Geometry: final body of the model. Coordinates: model frame, mm. Give positions to 0.01 mm unless a question says otherwise; leave off trailing zeros. Write each loop counter-clockwise with the first axis right and the second up, starting at its lowest first coordinate (ties: lowest second). Pieces come first, ordered by that corner, then holes.
Q1. Line query: line 1 (X direction, y = 195, z = 2); line 2 (X direction, y = 263.5, z = 4.75); line 3 (Y direction, x = 144.5, z = 3.25). Output: solid intervals per line, ascending.
Q2. Pin query (flat end, axial travel): pin 1 Ø0.8 at (x, y) = (144, 262.5) entering from -Z. Return the tip coordinate at first contact, or that it passes through.
Q3. Section A-A (x = 143.75). Return the cut outline in (y, z), plus the area to 3 significant figures.
Autodesk Inventor part; units mm, degrees
ref_plane "Work Plane1" through (146.6642, 216.5237, 7.3936) normal (0, 0, -1) x (0, 1, 0)
ref_plane "YZ Plane" through (0, 0, 0) normal (1, 0, 0) x (0, 1, 0)
ref_plane "XZ Plane" through (0, 0, 0) normal (0, 1, 0) x (-1, 0, 0)
sketch "Sketch1" plane through (0, 0, 0) normal (0, 0, 1) x (1, 0, 0)
  line L0 (165.7182, 252.0837) -> (146.6642, 252.0837)
  line L1 (158.6327, 216.5237) -> (165.7182, 216.5237)
  line L2 (139.5562, 216.5237) -> (143.6242, 216.5237)
  line L3 (143.6242, 252.0837) -> (139.5562, 252.0837)
  line L4 (126.4117, 267.0247) -> (136.1907, 267.0247)
  line L5 (136.1907, 190.8247) -> (126.4117, 190.8247)
  line L6 (139.5562, 267.0247) -> (139.5562, 190.8247)
  line L7 (139.5562, 190.8247) -> (165.7182, 190.8247)
  line L8 (165.7182, 190.8247) -> (165.7182, 267.0247)
  line L9 (165.7182, 267.0247) -> (139.5562, 267.0247)
  point P0 (0, 0)
ref_plane "Work Plane1" through (146.6642, 216.5237, 7.3936) normal (0, 0, -1) x (0, 1, 0)
extrude "Extrusion1" add sketch "Sketch1" along normal up to surface (7.3936 mm away)
fillet "Fillet1" radius 1 4 edges at (139.5562, 190.8247, 3.6968) (139.5562, 267.0247, 3.6968) (165.7182, 267.0247, 3.6968) (165.7182, 190.8247, 3.6968)
sketch "Sketch3" plane through (0, 0, 0) normal (0, 0, -1) x (-1, 0, 0)
  circle A0 centre (-160.3842, 185.8247) radius 1.25
  line L0 (-165.7182, 191.8247) -> (-165.7182, 194.8247)
  line L1 (-165.7182, 191.8247) -> (-165.7182, 266.0247)
  line L2 (-165.7182, 194.8247) -> (-161.7182, 194.8247)
  circle A1 centre (-161.7182, 194.8247) radius 1.25
  line L3 (-140.5562, 190.8247) -> (-164.7182, 190.8247)
  line L4 (-165.7182, 228.9247) -> (-156.0588, 228.9247)
  line L5 (-152.6372, 190.8247) -> (-152.6372, 206.7203)
  line L6 (-139.5562, 191.8247) -> (-139.5562, 194.8247)
  line L7 (-139.5562, 191.8247) -> (-139.5562, 266.0247)
  line L8 (-139.5562, 194.8247) -> (-143.5562, 194.8247)
  circle A2 centre (-143.5562, 194.8247) radius 1.25
  line L9 (-164.7182, 190.8247) -> (-140.5562, 190.8247)
  circle A3 centre (-160.3842, 272.0247) radius 1.25
  line L10 (-165.7182, 266.0247) -> (-165.7182, 263.0247)
  line L11 (-165.7182, 266.0247) -> (-165.7182, 191.8247)
  line L12 (-165.7182, 263.0247) -> (-161.7182, 263.0247)
  circle A4 centre (-161.7182, 263.0247) radius 1.25
  line L13 (-140.5562, 267.0247) -> (-164.7182, 267.0247)
  line L14 (-152.6372, 267.0247) -> (-152.6372, 251.1291)
  line L15 (-139.5562, 266.0247) -> (-139.5562, 263.0247)
  line L16 (-139.5562, 266.0247) -> (-139.5562, 191.8247)
  line L17 (-139.5562, 263.0247) -> (-143.5562, 263.0247)
  circle A5 centre (-143.5562, 263.0247) radius 1.25
  line L18 (-164.7182, 267.0247) -> (-140.5562, 267.0247)
  point P0 (0, 0)
  dimension "d11" = 3
  dimension "d12" = 4
  dimension "d13" = 2.5
  dimension "d14" = 4
extrude "Extrusion3" cut sketch "Sketch3" against normal blind 5 contours A4 | A1 | A5 | A2
properties part number "Supporter"
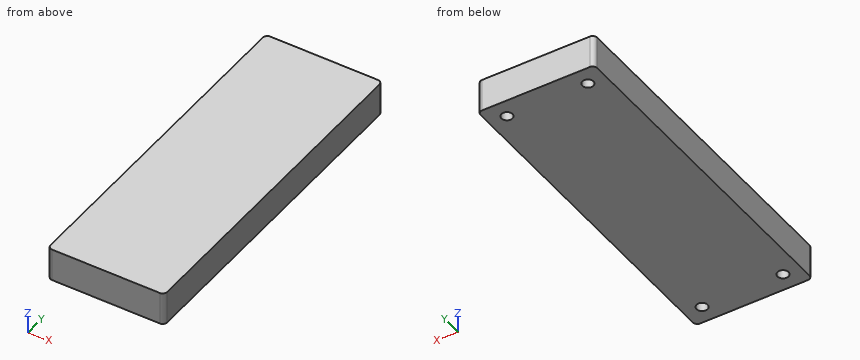
Computed:
1. line 1: x = 139.56 to 142.32, 144.79 to 160.48, 162.96 to 165.72
1. line 2: x = 139.56 to 142.4, 144.71 to 160.56, 162.87 to 165.72
1. line 3: y = 190.82 to 194.01, 195.64 to 262.21, 263.84 to 267.02
2. pin 1: stops at z = 5
3. outline: (190.82, 0) - (193.59, 0) - (193.59, 5) - (196.06, 5) - (196.06, 0) - (261.79, 0) - (261.79, 5) - (264.26, 5) - (264.26, 0) - (267.02, 0) - (267.02, 7.39) - (190.82, 7.39) - close
3. area: 539 mm2
